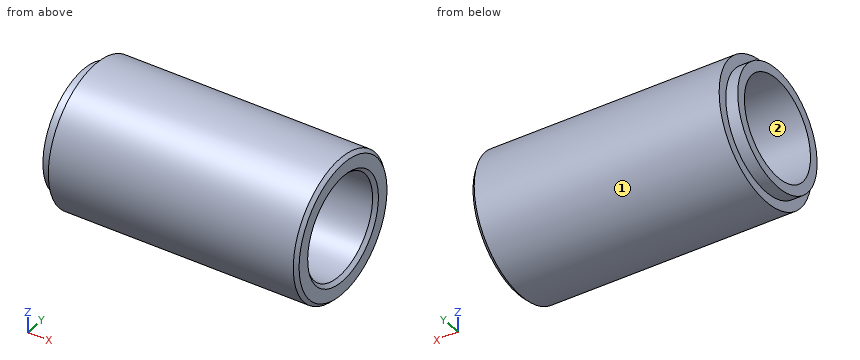
Autodesk Inventor part; units mm, degrees
ref_plane "YZ Plane" through (0, 0, 0) normal (1, 0, 0) x (0, 1, 0)
ref_plane "XZ Plane" through (0, 0, 0) normal (0, 1, 0) x (-1, 0, 0)
ref_plane "XY Plane" through (0, 0, 0) normal (0, 0, 1) x (1, 0, 0)
sketch "Skizze2" plane through (0, 0, 0) normal (0, 0, 1) x (1, 0, 0)
  line L0 (0, 0) -> (0, 6)
  line L1 (0, 6) -> (1.2, 6)
  line L2 (1.2, 6) -> (1.2, 7)
  line L3 (1.2, 7) -> (26, 7)
  line L4 (26, 7) -> (26, 0)
  line L5 (26, 0) -> (0, 0)
  dimension "d0" = 26
  dimension "d1" = 14
  dimension "d2" = 12
  dimension "d3" = 1.2
revolve "Umdrehung1" add sketch "Skizze2" angle 360 about axis through (26, 0, 0) along (-1, 0, 0)
sketch "Skizze3" plane through (0, 0, 0) normal (-1, 0, 0) x (0, 0, 1)
  circle A0 centre (0, 0) radius 5
  dimension "d5" = 10
extrude "Extrusion1" cut sketch "Skizze3" against normal up to surface (26 mm away)
chamfer "Fasen1" distance 0.35 angle 45 2 edges at (26, 0, -5) (26, -7, 0)
properties part number "Ak zylinder" material "Messing, weicher Gelbton, geschweißt"
Source: CAD feature listing. Evaluate the final solid. Frame: model axes, mm. Face numbers are marked on the shaded views. Coordinates: 2 decimals unless noted, no trailing zeros. Loops run counter-clockwise (first coordinate to the right, second up) from the corner with the lowest first, then second, coordinate; pieces in that order, holes last. Notation, with made-up numbers: M 89.5,-28 L 121.5,-28 A23 ccw 121.5,-20 Z; hole C 80.25,-11.75 d9. An arc over 180 degrees is marked long. Put each result on its own line as item: value. Start each with the question number.
1) Cut plane C-C on x = 5.5. Return the cut outline in (y, z).
2) Pull-direction query (Z, two-part tool) for the marked faces 1 and 2; classes: pulls with the +Z half, pulls with the -Z half, needs draft (parallel to the pull), parting line crosses it, or undercut.
3) Ray query, L1, parallel to Z at x = 1.5, y = -0.25; L2, parallel to Y at x = 18.5, z = 0; L3, parallel to Z at x = 24.25, y = -0.75. Return the intervals inside material, ascending. Write a range as from..to.
4) Contact query for flat-ended pins moving along their axis: pin 1 Ø1 at (x, z) = (19, 3) entering from -Y; pin 2 Ø8 at (y, z) = (0, 0) entering from -X; pin 3 Ø1.5 at (x, y) = (9.5, 1) entering from +Z; pin 4 Ø2 at (y, z) = (5, 5) entering from -X. Output: stop coordinate, or through.
5) Cut plane A-A on z = 0. Return the cut outline in (x, y).
The answers:
1. outline: C 0,0 d14; hole C 0,0 d10
2. face 1: parting line crosses it
2. face 2: undercut
3. L1: z = -7..-4.99, 4.99..7
3. L2: y = -7..-5, 5..7
3. L3: z = -6.96..-4.94, 4.94..6.96
4. pin 1: stops at y = -6.54
4. pin 2: passes through
4. pin 3: stops at z = 7
4. pin 4: stops at x = 1.2
5. outline: M 0,-6 L 1.2,-6 L 1.2,-7 L 25.65,-7 L 26,-6.65 L 26,-5.35 L 25.65,-5 L 0,-5 Z; M 0,5 L 25.65,5 L 26,5.35 L 26,6.65 L 25.65,7 L 1.2,7 L 1.2,6 L 0,6 Z
